Part model, mm, in its own coordinate system. A direction names the side the tool comes from. Coordinates: 2 decimals unless noted, no trailing zeros. Loops run counter-clockwise (first coordinate to the right, second up) from the corner with the lowest first, then second, coordinate; pieces in that order, holes last. Notation, with made-up numbers: (58, 6.25) - (104, 6.25) arc R10 cw to (104, 17.25) - close; hole circle Ø11 at (73.25, 68.5). An arc over 180 degrees is marked (long way). Use a Markdown table: item, result. Add a question column.
1) Probe probe 1 along X at (y, z) = (673.5, 91.5); probe 2 along Z at (x, y) = (90, 682.25); probe 3 along X at (y, z) = (677, 94). List the from-to ranges inside material, lowest first. Write a range as [from, to].
2) Band-saw the part on B-B (z = 111.5). Give the cut face in (x, y) (3 decimals).
3) Drop flat-ended pins along their axis: P1, Ø5, axis at x = 115, y = 679, coming from the -Z side; P2, Ø4, axis at x = 110, z = 56.5, coming from the +Y side; P3, Ø7.5, axis at x = 93.07, z = 91.5, coming from the -Y side; P4, Ø7.5, axis at x = 93.07, z = 91.5, coming from the +Y side. Give the stop position or say it passes through.
4) Band-saw the part on C-C (x = 128.5). Give the cut face in (y, z), plus the area to 3 significant figures.
5) Pull direction Z, two halves, no side cores. Call faces 1 (the face through (118.567, 673, 86)), 2 (the face through (134.867, 679, 59)): +Z half, -Z half, draft (parallel to the pull), parting line (faces both ways), or undercut.
6) Tool access for faces 3 (the face through (110.9, 672.5, 99.5)), 4 (the face through (96, 679.043, 92)), 5 (the face through (123.45, 680.11, 58.67)): list every direction of +Z, -Z, +X, -X, +Y, -Y with a clear straight run to the whole face (end or side of a thin tool).
7) Band-saw the part on D-D (y = 680.75). Give the cut face in (x, z) (3 decimals).
8) Band-saw the part on A-A (y = 671.75). Give the cut face in (x, z), plus the area to 3 significant figures.
from build123d import *

# Parameters (mm, degrees)
EXTRUDE_1_DEPTH     = 119
SKETCH_4_R          = 4.145
CUT_EXTRUDE_2_DEPTH = 5
SKETCH_7_R          = 2.8
CUT_EXTRUDE_3_DEPTH = 10
CUT_EXTRUDE_4_DEPTH = 10


with BuildPart() as part:
    # 草图1 → 凸台-拉伸1 (new body)
    with BuildSketch(Plane.XY):
        Polygon((100.067060811, 682.684424639), (88.767060811, 682.684424639), (88.087771489, 683.363713961), (88.767060811, 684.043003282), (98.708482167, 684.043003282), align=None)
        Polygon((88.767060811, 682.684424639), (88.767060811, 670.543003282), (87.767060811, 669.543003282), (87.267060811, 670.043003282), (87.267060811, 682.543003282), (88.087771489, 683.363713961), align=None)
        with BuildLine():
            ThreePointArc((100.067060811, 682.308234217), (98.682060811, 680.143003282), (100.067060811, 677.977772348))
            Line((100.067060811, 677.977772348), (100.067060811, 676.343003282))
            ThreePointArc((100.067060811, 676.343003282), (100.301375386, 675.777317857), (100.867060811, 675.543003282))
            Line((100.867060811, 675.543003282), (121.267060811, 675.543003282))
            ThreePointArc((121.267060811, 675.543003282), (121.832746236, 675.777317857), (122.067060811, 676.343003282))
            Line((122.067060811, 676.343003282), (122.067060811, 677.977772348))
            ThreePointArc((122.067060811, 677.977772348), (123.452060811, 680.143003282), (122.067060811, 682.308234217))
            Line((122.067060811, 682.308234217), (122.067060811, 682.684424639))
            Line((122.067060811, 682.684424639), (133.367060811, 682.684424639))
            Line((133.367060811, 682.684424639), (133.367060811, 670.543003282))
            Line((133.367060811, 670.543003282), (88.767060811, 670.543003282))
            Line((88.767060811, 670.543003282), (88.767060811, 682.684424639))
            Line((88.767060811, 682.684424639), (100.067060811, 682.684424639))
            Line((100.067060811, 682.684424639), (100.067060811, 682.308234217))
        make_face()
        Polygon((88.767060811, 670.543003282), (133.367060811, 670.543003282), (134.367060811, 669.543003282), (133.867060811, 669.043003282), (121.567060811, 669.043003282), (121.217060811, 669.393003282), (100.917060811, 669.393003282), (100.567060811, 669.043003282), (88.267060811, 669.043003282), (87.767060811, 669.543003282), align=None)
        Polygon((133.367060811, 682.684424639), (122.067060811, 682.684424639), (123.425639455, 684.043003282), (123.667060811, 684.043003282), (133.367060811, 684.043003282), (134.046350133, 683.363713961), align=None)
        with BuildLine():
            ThreePointArc((134.867060811, 676.243003282), (134.330385769, 675.243003282), (134.867060811, 674.243003282))
            Line((134.867060811, 674.243003282), (134.867060811, 670.043003282))
            Line((134.867060811, 670.043003282), (134.367060811, 669.543003282))
            Line((134.367060811, 669.543003282), (133.367060811, 670.543003282))
            Line((133.367060811, 670.543003282), (133.367060811, 682.684424639))
            Line((133.367060811, 682.684424639), (134.046350133, 683.363713961))
            Line((134.046350133, 683.363713961), (134.867060811, 682.543003282))
            Line((134.867060811, 682.543003282), (134.867060811, 676.243003282))
        make_face()
    extrude(amount=EXTRUDE_1_DEPTH)

    # 草图4 → 切除-拉伸2 (cut)
    with BuildSketch(Plane(origin=(0, 684.043003282, 0), x_dir=(1, 0, 0), z_dir=(0, 1, 0))):
        with Locations((93.067060811, -27.5)):
            Circle(SKETCH_4_R)
        with Locations((129.067060811, -27.5)):
            Circle(SKETCH_4_R)
        with Locations((93.067060811, -91.5)):
            Circle(SKETCH_4_R)
        with Locations((129.067060811, -91.5)):
            Circle(SKETCH_4_R)
    extrude(amount=-CUT_EXTRUDE_2_DEPTH, mode=Mode.SUBTRACT)

    # 草图7 → 切除-拉伸3 (cut)
    with BuildSketch(Plane(origin=(0, 679.043003282, 0), x_dir=(1, 0, 0), z_dir=(0, 1, 0))):
        with Locations((93.067060811, -27.5)):
            Circle(SKETCH_7_R)
        with Locations((93.067060811, -91.5)):
            Circle(SKETCH_7_R)
        with Locations((129.067060811, -91.5)):
            Circle(SKETCH_7_R)
        with Locations((129.067060811, -27.5)):
            Circle(SKETCH_7_R)
    extrude(amount=-CUT_EXTRUDE_3_DEPTH, mode=Mode.SUBTRACT)

    # 草图8 → 切除-拉伸4 (cut)
    with BuildSketch(Plane(origin=(0, 675.543003282, 0), x_dir=(1, 0, 0), z_dir=(0, 1, 0))):
        with BuildLine():
            Line((103.567060811, -27), (103.567060811, -40))
            ThreePointArc((103.567060811, -40), (111.067060811, -47.5), (118.567060811, -40))
            Line((118.567060811, -40), (118.567060811, -27))
            ThreePointArc((118.567060811, -27), (111.067060811, -19.5), (103.567060811, -27))
        make_face()
        with BuildLine():
            Line((103.567060811, -79), (103.567060811, -92))
            ThreePointArc((103.567060811, -92), (111.067060811, -99.5), (118.567060811, -92))
            Line((118.567060811, -92), (118.567060811, -79))
            ThreePointArc((118.567060811, -79), (111.067060811, -71.5), (103.567060811, -79))
        make_face()
    extrude(amount=-CUT_EXTRUDE_4_DEPTH, mode=Mode.SUBTRACT)


solid = part.part
Answer block:
| question | item | result |
|---|---|---|
| 1 | probe 1 | [87.27, 90.27], [95.87, 103.57], [118.57, 126.27], [131.87, 134.87] |
| 1 | probe 2 | [0, 24.71], [30.29, 88.71], [94.29, 119] |
| 1 | probe 3 | [87.27, 91.81], [94.33, 100.07], [122.07, 127.81], [130.33, 134.87] |
| 2 | outline | (87.267, 670.043) - (88.267, 669.043) - (100.567, 669.043) - (100.917, 669.393) - (121.217, 669.393) - (121.567, 669.043) - (133.867, 669.043) - (134.867, 670.043) - (134.867, 674.243) arc R1.2 cw to (134.867, 676.243) - (134.867, 682.543) - (133.367, 684.043) - (123.426, 684.043) - (122.067, 682.684) - (122.067, 682.308) arc R2.385 cw to (122.067, 677.978) - (122.067, 676.343) arc R0.8 cw to (121.267, 675.543) - (100.867, 675.543) arc R0.8 cw to (100.067, 676.343) - (100.067, 677.978) arc R2.385 cw to (100.067, 682.308) - (100.067, 682.684) - (98.708, 684.043) - (88.767, 684.043) - (87.267, 682.543) - close |
| 3 | P1 | through |
| 3 | P2 | y = 675.54 |
| 3 | P3 | y = 669.04 |
| 3 | P4 | y = 679.04 |
| 4 | outline | (669.04, 0) - (684.04, 0) - (684.04, 23.39) - (679.04, 23.39) - (679.04, 24.76) - (669.04, 24.76) - close; (669.04, 30.24) - (679.04, 30.24) - (679.04, 31.61) - (684.04, 31.61) - (684.04, 87.39) - (679.04, 87.39) - (679.04, 88.76) - (669.04, 88.76) - close; (669.04, 94.24) - (679.04, 94.24) - (679.04, 95.61) - (684.04, 95.61) - (684.04, 119) - (669.04, 119) - close |
| 4 | area | 1,590 mm2 |
| 5 | face 1 | undercut |
| 5 | face 2 | draft |
| 6 | face 3 | +Y, -Y |
| 6 | face 4 | +Y |
| 6 | face 5 | +Z, -Z |
| 7 | outline | (87.267, 0) - (98.761, 0) - (98.761, 119) - (87.267, 119) - close; (123.374, 0) - (134.867, 0) - (134.867, 119) - (123.374, 119) - close; hole circle Ø8.29 at (93.067, 27.5); hole circle Ø8.29 at (93.067, 91.5); hole circle Ø8.29 at (129.067, 27.5); hole circle Ø8.29 at (129.067, 91.5) |
| 8 | outline | (87.27, 0) - (134.87, 0) - (134.87, 119) - (87.27, 119) - close; hole circle Ø5.6 at (93.07, 27.5); hole circle Ø5.6 at (93.07, 91.5); hole (103.57, 27) arc R7.5 ccw to (118.57, 27) - (118.57, 40) arc R7.5 ccw to (103.57, 40) - close; hole (103.57, 79) arc R7.5 ccw to (118.57, 79) - (118.57, 92) arc R7.5 ccw to (103.57, 92) - close; hole circle Ø5.6 at (129.07, 27.5); hole circle Ø5.6 at (129.07, 91.5) |
| 8 | area | 4,820 mm2 |
